```python
from build123d import *

# Parameters (mm, degrees)
CUT_EXTRUDE_1_REACH = 28.824
SKETCH_1_R          = 11.30959092
CUT_EXTRUDE_2_REACH = 28.261
SKETCH_2_R          = 2.7


with BuildPart() as part:
    # Sketch1 → Revolve1 (revolve)
    with BuildSketch(Plane.XY, mode=Mode.PRIVATE) as revolve1_sk:
        Polygon((11.15, 18.5), (5.082863863, 18.5), (5.082863863, 20), (11.15, 20), (11.15, 21), (4.951844414, 21), (4.951844414, 22.5), (11.15, 22.5), (11.15, 23.5), (4.820824966, 23.5), (4.820824966, 25), (11.15, 25), (11.15, 26), (4.689805518, 26), (4.689805518, 27.5), (8, 27.5), (8, 28.5), (4.689805518, 28.5), (4.689805518, 30), (8, 30), (8, 33), (6, 33), (6, 39), (8, 39), (8, 42.7), (4, 42.7), (4, 36.6), (2.1, 34.7), (2.1, 14.7), (3.5, 13.3), (3.5, 0), (11.15, 0), (11.15, 1), (6, 1), (6, 2.5), (11.15, 2.5), (11.15, 3.5), (5.868980552, 3.5), (5.868980552, 5), (11.15, 5), (11.15, 6), (5.737961104, 6), (5.737961104, 7.5), (11.15, 7.5), (11.15, 8.5), (5.606941655, 8.5), (5.606941655, 10), (11.15, 10), (11.15, 11), (5.475922207, 11), (5.475922207, 12.5), (11.15, 12.5), (11.15, 13.5), (5.344902759, 13.5), (5.344902759, 15), (11.15, 15), (11.15, 16), (5.213883311, 16), (5.213883311, 17.5), (11.15, 17.5), align=None)
    revolve(revolve1_sk.sketch.rotate(Axis((0, 42.7, 0), (0, -1, 0)), 270), axis=Axis((0, 42.7, 0), (0, -1, 0)))

    # Эскиз1 → Вырез-Вытянуть1 (cut, up to next)
    with BuildSketch(Plane(origin=(0, 21, 0), x_dir=(1, 0, 0), z_dir=(0, 1, 0)), mode=Mode.PRIVATE) as cut_extrude_1_sk1:
        Circle(SKETCH_1_R)
    cut_extrude_1_tool1 = extrude(cut_extrude_1_sk1.sketch, amount=CUT_EXTRUDE_1_REACH, mode=Mode.PRIVATE) & part.part
    add(cut_extrude_1_tool1.solids().sort_by_distance((0, 21, 0))[0], mode=Mode.SUBTRACT)

    # Вырез-Вытянуть2: up to this cone (the profile starts outside it)
    cut_extrude_2_end = Plane(origin=(0, 21, 0), z_dir=(0, -1, 0)).offset(4.200001) * Cone(1e-06, 24.561, 24.560999, align=(Align.CENTER, Align.CENTER, Align.MIN), mode=Mode.PRIVATE)
    # Эскиз2 → Вырез-Вытянуть2 (cut, up to the surface)
    with BuildSketch(Plane(origin=(0, 21, 0), x_dir=(1, 0, 0), z_dir=(0, 1, 0)), mode=Mode.PRIVATE) as cut_extrude_2_sk1:
        with Locations(Location((0, 0, 0), (0, 0, 270))):
            Circle(SKETCH_2_R)
    cut_extrude_2_tool1 = extrude(cut_extrude_2_sk1.sketch, amount=-CUT_EXTRUDE_2_REACH, mode=Mode.PRIVATE) - cut_extrude_2_end
    add(cut_extrude_2_tool1.solids().sort_by_distance((0, 21, 0))[0], mode=Mode.SUBTRACT)


solid = part.part
```
Here's how the part is built. I have some questions about the finished solid (model axes, mm). A direction names the side the tool comes from. Coordinates: 2 decimals unless noted, no trailing zeros. Answer as CSV lines item,"result".
Q1. For pin 1 (1.5 mm diameter, centred on x = -1.5, y = 12.5, fed in from +Z); pin 2 (2 mm diameter, centred on y = 8.5, z = 4.5, fed in from -X); pin 3 (8 mm diameter, centred on y = 19, z = 7.5, fed in from +X), each with a flat end and sliding along its axis, tell me the tip position at first contact or that it passes through.
Response:
pin 1,"z = 11.12"
pin 2,"x = -10.59"
pin 3,"x = 10.58"
Q2. For faces 1 (the face through (-5, 16, -2)), 2 (the face through (-3.417, 6.557, 0.759)), 3 (the face through (-10.885, 18.007, 2.417)), which set-ups out of +Z, -Z, +X, -X, +Y, -Y let a thin tool reach every point of the face, with its end or its side?
Response:
face 1,"none"
face 2,"-Y"
face 3,"+Y, -Y"
Q3. We'd pull the mould along Y, two halves only. Please class faces 4 (the face through (-10.885, 8.007, 2.417)), 5 (the face through (1.802, 1.76, -5.723)), 6 (the face through (4.286, 19.26, -2.733)), 7 (the face through (3, 0, -3)): pulls with the +Y half, pulls with the -Y half, needs draft (parallel to the pull), parting line crosses it, or undercut.
Response:
face 4,"needs draft"
face 5,"undercut"
face 6,"undercut"
face 7,"pulls with the -Y half"
Q4. If I drill on L1, parallel to X at y = 3, z = 0; L2, parallel to X at y = 4.25, z = 0; L3, parallel to Z at x = -3, y = 3, over which ranges is the centre line in solid material (lowest first)? Write a range as [from, to].
Response:
L1,"[-11.15, -3.5], [3.5, 11.15]"
L2,"[-5.87, -3.5], [3.5, 5.87]"
L3,"[-10.74, -1.8], [1.8, 10.74]"
Q5. If we section it at A-A, the plane x = 7.75: Give the number of separate pieces and of enclosed holes in the cut face, and give its area (3 significant figures).
Response:
separate pieces,"9"
enclosed holes,"0"
area,"144 mm2"
